```python
from build123d import *

# Parameters (mm, degrees)
SKETCH5_R                        = 7.5
SKETCH5_R_2                      = 5.5
EXTRUDE_THIN5_DEPTH              = 3.5
SKETCH6_R                        = 6.5
BOSS_EXTRUDE1_DEPTH              = 28.5
F_11_5_11_5_DIAMETER_HOLE1_D     = 11.5
F_11_5_11_5_DIAMETER_HOLE1_DEPTH = 18.5
F_11_5_11_5_DIAMETER_HOLE1_TIP   = 3.592998773
F_11_0_11_DIAMETER_HOLE2_D       = 11
F_11_0_11_DIAMETER_HOLE2_DEPTH   = 4
F_11_0_11_DIAMETER_HOLE2_TIP     = 3.436781436


with BuildPart() as part:
    # Sketch5 → Extrude-Thin5 (new body)
    with BuildSketch(Plane(origin=(0, 0, 0), x_dir=(1, 0, 0), z_dir=(0, 1, 0))):
        Circle(SKETCH5_R)
        Circle(SKETCH5_R_2, mode=Mode.SUBTRACT)
    extrude(amount=-EXTRUDE_THIN5_DEPTH)

    # Sketch6 → Boss-Extrude1 (add)
    with BuildSketch(Plane(origin=(0, 0, 0), x_dir=(1, 0, 0), z_dir=(0, 1, 0))):
        Circle(SKETCH6_R)
    extrude(amount=BOSS_EXTRUDE1_DEPTH)

    # Ø11.5 (11.5) Diameter Hole1
    with Locations(Plane.ZX.offset(28.5)):
        with Locations((0, 0)):
            Hole(F_11_5_11_5_DIAMETER_HOLE1_D / 2, depth=F_11_5_11_5_DIAMETER_HOLE1_DEPTH)
            with Locations((0, 0, -(F_11_5_11_5_DIAMETER_HOLE1_DEPTH + F_11_5_11_5_DIAMETER_HOLE1_TIP / 2))):  # 116° drill point
                Cone(0, F_11_5_11_5_DIAMETER_HOLE1_D / 2, F_11_5_11_5_DIAMETER_HOLE1_TIP, mode=Mode.SUBTRACT)

    # Ø11.0 (11) Diameter Hole2
    with Locations(Plane(origin=(0, -3.5, 0), x_dir=(0, 0, -1), z_dir=(0, -1, 0))):
        with Locations((0, 0)):
            Hole(F_11_0_11_DIAMETER_HOLE2_D / 2, depth=F_11_0_11_DIAMETER_HOLE2_DEPTH)
            with Locations((0, 0, -(F_11_0_11_DIAMETER_HOLE2_DEPTH + F_11_0_11_DIAMETER_HOLE2_TIP / 2))):  # 116° drill point
                Cone(0, F_11_0_11_DIAMETER_HOLE2_D / 2, F_11_0_11_DIAMETER_HOLE2_TIP, mode=Mode.SUBTRACT)


solid = part.part
```
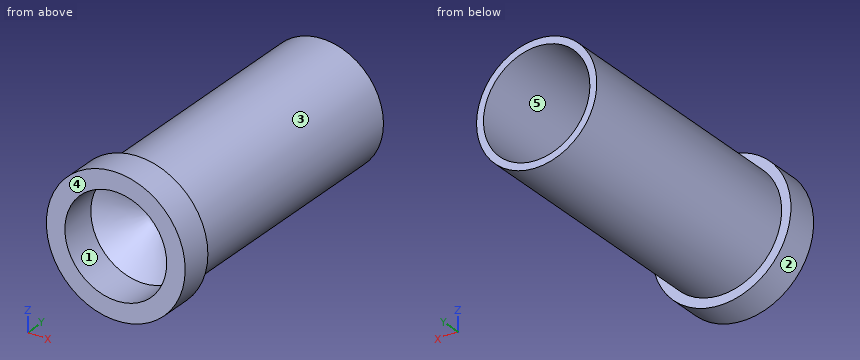
Check sheet for the modelled part. Datum: model origin and axes. Units: mm. Face numbers are marked on the shaded views. A direction names the side the tool comes from. Coordinates: 2 decimals unless noted, no trailing zeros. Write each loop counter-clockwise with the first axis right and the second up, starting at its lowest first coordinate (ties: lowest second). Pieces come first, ordered by that corner, then holes. Notation, with made-up numbers: (13, 86) - (35, 86) arc R28 cw to (35, 117) - close; hole circle Ø3 at (60.5, -10). An arc over 180 degrees is marked (long way). One line per question, with ' | ' between items.
Item 1: Access from +Z, -Z, +X, -X, +Y, -Y to the whole of each face (thin tool, end or side, straight path). Record for the marked faces 1 and 2.
Determined:
face 1: -Y | face 2: +Y, -Y
Item 2: Sectioned sample at A-A on y = 21. Record the boundary of the cut face in (x, z).
Determined:
outline: circle Ø13 at (0, 0); hole circle Ø11.5 at (0, 0)
Item 3: Sectioned sample at B-B on y = 4.5. Record the boundary of the cut face in (x, z), plus the area to 3 significant figures.
Determined:
outline: circle Ø13 at (0, 0) | area: 133 mm2
Item 4: Gauge pin test, flat ends, axial feed: P1, Ø3, axis at x = -2, z = 0.5, coming from the -Y side; P2, Ø3, axis at y = 20.5, z = -2, coming from the +X side; P3, Ø4, axis at x = 5.5, y = 9, coming from the -Z side. Record the tip position at first contact, or that the pin passes through.
Determined:
P1: stops at y = 1.71 | P2: stops at x = 6.48 | P3: stops at z = -5.48
Item 5: Thickness scan on line 1 (Z direction, x = 0, y = -0.7); line 2 (Z direction, x = 0, y = 22); line 3 (X direction, y = 17.5, z = 2.5). Record the ranges inside material, lowest first. Write a range as [from, to].
Determined:
line 1: z = [-7.5, -5.5], [5.5, 7.5] | line 2: z = [-6.5, -5.75], [5.75, 6.5] | line 3: x = [-6, -5.18], [5.18, 6]
Item 6: Mould release check, pull along X, two halves, no side actions. Record for the marked faces 3, 4 and 5: pulls with the +X half, pulls with the -X half, needs draft (parallel to the pull), parting line crosses it, or undercut.
Determined:
face 3: parting line crosses it | face 4: needs draft | face 5: undercut
